Part print with two shaded views. Sizes in mm from the minimum x, y, z corner. A direction names the side the tool comes from. Give positions to 0.01 mm unless a question says otherwise; leave off trailing zeros. Order: outer loops, then holes, each group sorted by start corner. A loop starts at its lowest first (then second) coordinate and runs counter-clockwise, first axis right, second up. Notation, with made-up numbers: M 5,83.25 L 60,83.25 A7 cw 60,90.25 Z; hole C -4,-38.75 d1. An arc over 180 degrees is marked long. Answer as CSV lines item,"result".
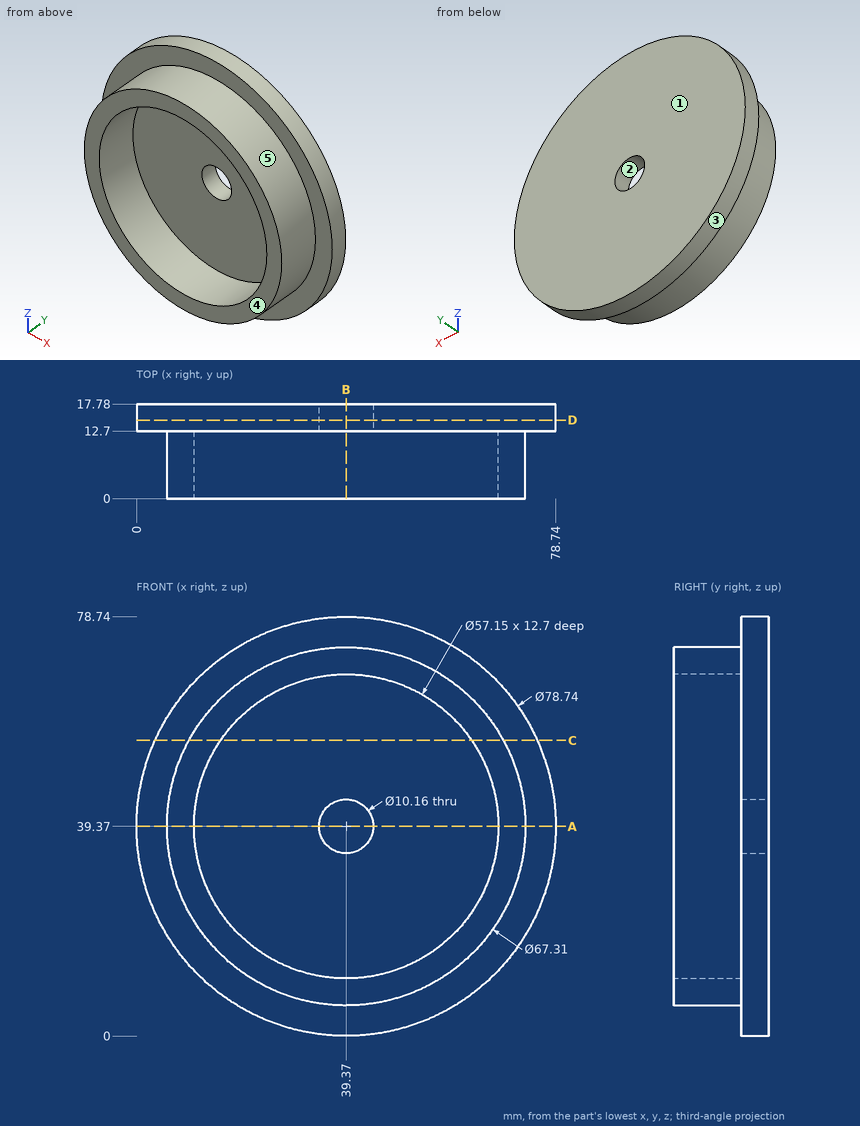
Item 1: Probe line 1 along X through (y, z) = (10, 39.37) (3 decimals); line 2 along Z through (x, y) = (39.37, 14). List the from-to ranges inside material, lowest first. Write a range as from..to.
Geometry says:
line 1,"x = 5.715..10.795, 67.945..73.025"
line 2,"z = 0..34.29, 44.45..78.74"
Item 2: Pull direction X, two halves, no side cores. Call the marked faces 1, 2 and 3: released by +X, released by -X, zero draft, split by the parting line, or undercut.
Geometry says:
face 1,"zero draft"
face 2,"undercut"
face 3,"split by the parting line"
Item 3: Band-saw the part on A-A (z = 39.37). Give the cut face in (x, y) (3 decimals).
Geometry says:
outline,"M 0,12.7 L 5.715,12.7 L 5.715,0 L 10.795,0 L 10.795,12.7 L 34.29,12.7 L 34.29,17.78 L 0,17.78 Z; M 44.45,12.7 L 67.945,12.7 L 67.945,0 L 73.025,0 L 73.025,12.7 L 78.74,12.7 L 78.74,17.78 L 44.45,17.78 Z"
Item 4: Band-saw the part on C-C (z = 55.5). Give the cut face in (x, y), and give its area (3 significant figures).
Geometry says:
outline,"M 3.46,12.7 L 9.83,12.7 L 9.83,0 L 15.78,0 L 15.78,12.7 L 62.96,12.7 L 62.96,0 L 68.91,0 L 68.91,12.7 L 75.28,12.7 L 75.28,17.78 L 3.46,17.78 Z"
area,"516 mm2"
Item 5: Drop flat-ended pins along their axis: pin 1 (1 mm diameter, centred on x = 9, y = 14, fed in from +Z); pin 2 (5 mm diameter, centred on x = 38.5, y = 2, fed in from +Z) (3 decimals); pin 3 (3 mm diameter, centred on x = 15, y = 14, fed in from -Z). Give the stop position or say it passes through.
Geometry says:
pin 1,"stops at z = 65.02"
pin 2,"stops at z = 73.025"
pin 3,"stops at z = 7.32"
Item 6: Band-saw the part on B-B (x = 39.37). Give the cut face in (y, z) (3 decimals).
Geometry says:
outline,"M 0,5.715 L 12.7,5.715 L 12.7,0 L 17.78,0 L 17.78,34.29 L 12.7,34.29 L 12.7,10.795 L 0,10.795 Z; M 0,67.945 L 12.7,67.945 L 12.7,44.45 L 17.78,44.45 L 17.78,78.74 L 12.7,78.74 L 12.7,73.025 L 0,73.025 Z"
Item 7: 3-axis set-ups, long thin cutter, end or side, ignore diameter. For the marked faces 4 and 5: which of +Z, -Z, +X, -X, +Y, -Y reach the whole face in a straight line?
Geometry says:
face 4,"+Z, -Z, +X, -X, -Y"
face 5,"-Y"
Item 8: Band-saw the part on D-D (y = 14.75). Give the cut face in (x, z), and give its area (3 significant figures).
Geometry says:
outline,"C 39.37,39.37 d78.74; hole C 39.37,39.37 d10.16"
area,"4,790 mm2"
